from build123d import *

# Parameters (mm, degrees)
PAD_DEPTH       = 70
POCKET_DEPTH    = 22
SKETCH008_W     = 61.659011
SKETCH008_H     = 41.462551
SKETCH008_W_2   = 60.331963
SKETCH008_H_2   = 13.684097
POCKET001_DEPTH = 76
SKETCH003_R     = 1.9
POCKET002_DEPTH = 12
POCKET003_DEPTH = 4
POCKET004_DEPTH = 6
SKETCH009_R     = 1.35
POCKET005_DEPTH = 10
SKETCH030_W     = 28.769002
SKETCH030_H     = 32
POCKET006_DEPTH = 48.001
SKETCH031_W     = 46.619307
SKETCH031_H     = 35.048725
POCKET007_DEPTH = 36
SKETCH032_R     = 1.9
POCKET008_DEPTH = 10
SKETCH013_R     = 1.9
POCKET009_DEPTH = 16
SKETCH010_R     = 1.6
POCKET010_DEPTH = 7
POCKET011_DEPTH = 60.501
POCKET012_DEPTH = 12.001
FILLET_R        = 3
CHAMFER_SIZE    = 3
FILLET001_R     = 5
FILLET002_R     = 9
FILLET003_R     = 0.7
FILLET004_R     = 1
FILLET005_R     = 1
FILLET006_R     = 3
FILLET007_R     = 1
FILLET008_R     = 1
CHAMFER001_SIZE = 13
FILLET009_R     = 1
FILLET010_R     = 16


with BuildPart() as part:
    # Sketch → Pad (new body)
    with BuildSketch(Plane.XY):
        Polygon((0, 0), (44, 0), (44, -60.5), (-14, -60.5), (-14, 0), align=None)
    extrude(amount=PAD_DEPTH)

    # Sketch002 (on Face7 of Pad) → Pocket (cut)
    with BuildSketch(Plane.XY.offset(70)):
        Polygon((32, -6), (32, -65.096024), (-40.783405, -65.096024), (-40.783405, 12.994774), (20, 12.994774), (20, -6), align=None)
    extrude(amount=-POCKET_DEPTH, mode=Mode.SUBTRACT)

    # Sketch008 (on Face3 of Pocket) → Pocket001 (cut)
    with BuildSketch(Plane.YZ.offset(44)):
        with Locations((-36.829505, -1.731275)):
            Rectangle(SKETCH008_W, SKETCH008_H)
        with Locations((-36.165982, 66.842049)):
            Rectangle(SKETCH008_W_2, SKETCH008_H_2)
    extrude(amount=-POCKET001_DEPTH, mode=Mode.SUBTRACT)

    # Sketch003 (on Face6 of Pocket001) → Pocket002 (cut)
    with BuildSketch(Plane.XY.offset(48)):
        with Locations((0, -13)):
            Circle(SKETCH003_R)
        with Locations((0, -57)):
            Circle(SKETCH003_R)
    extrude(amount=-POCKET002_DEPTH, mode=Mode.SUBTRACT)

    # Sketch004 (on Face6 of Pocket002) → Pocket003 (cut)
    with BuildSketch(Plane.XY.offset(48)):
        with BuildLine():
            ThreePointArc((0, -43.125), (8.125, -35), (0, -26.875))
            Line((-25, -26.875), (0, -26.875))
            Line((-25, -43.125), (-25, -26.875))
            Line((0, -43.125), (-25, -43.125))
        make_face()
    extrude(amount=-POCKET003_DEPTH, mode=Mode.SUBTRACT)

    # Sketch018 (on Face22 of Pocket003) → Pocket004 (cut)
    with BuildSketch(Plane.XY.offset(44)):
        with BuildLine():
            ThreePointArc((0, -41.1), (6.1, -35), (0, -28.9))
            Line((0, -28.9), (-50, -28.9))
            Line((-50, -41.1), (-50, -28.9))
            Line((0, -41.1), (-50, -41.1))
        make_face()
    extrude(amount=-POCKET004_DEPTH, mode=Mode.SUBTRACT)

    # Sketch009 (on Face3 of Pocket004) → Pocket005 (cut)
    with BuildSketch(Plane.YZ.offset(44)):
        with Locations((-44, 55)):
            Circle(SKETCH009_R)
        with Locations((-13, 24)):
            Circle(SKETCH009_R)
        with Locations((-13, 55)):
            Circle(SKETCH009_R)
        with Locations((-44, 24)):
            Circle(SKETCH009_R)
    extrude(amount=-POCKET005_DEPTH, mode=Mode.SUBTRACT)

    # Sketch030 (on Face6 of Pocket005) → Pocket006 (cut, through all)
    with BuildSketch(Plane.XY.offset(48)):
        with Locations((-14.384501, -35)):
            Rectangle(SKETCH030_W, SKETCH030_H)
    extrude(amount=-POCKET006_DEPTH, mode=Mode.SUBTRACT)

    # Sketch031 (on Face8 of Pocket006) → Pocket007 (cut)
    with BuildSketch(Plane(origin=(-14, 0, 0), x_dir=(0, -1, 0), z_dir=(-1, 0, 0))):
        with Locations((29.409654, 20.475638)):
            Rectangle(SKETCH031_W, SKETCH031_H)
    extrude(amount=-POCKET007_DEPTH, mode=Mode.SUBTRACT)

    # Sketch032 (on Face8 of Pocket007) → Pocket008 (cut)
    with BuildSketch(Plane(origin=(-14, 0, 0), x_dir=(0, -1, 0), z_dir=(-1, 0, 0))):
        with Locations((12, 44)):
            Circle(SKETCH032_R)
        with Locations((55, 44)):
            Circle(SKETCH032_R)
    extrude(amount=-POCKET008_DEPTH, mode=Mode.SUBTRACT)

    # Sketch013 (on Face21 of Pocket008) → Pocket009 (cut)
    with BuildSketch(Plane(origin=(0, 0, 0), x_dir=(0, -1, 0), z_dir=(-1, 0, 0))):
        with Locations((24, 42)):
            Circle(SKETCH013_R)
        with Locations((46, 42)):
            Circle(SKETCH013_R)
    extrude(amount=-POCKET009_DEPTH, mode=Mode.SUBTRACT)

    # Sketch010 (on Face1 of Pocket009) → Pocket010 (cut)
    with BuildSketch(Plane(origin=(0, 0, 0), x_dir=(-1, 0, 0), z_dir=(0, 1, 0))):
        with Locations((-32, 5)):
            Circle(SKETCH010_R)
        with Locations((-39, 65)):
            Circle(SKETCH010_R)
        with Locations((-25, 65)):
            Circle(SKETCH010_R)
    extrude(amount=-POCKET010_DEPTH, mode=Mode.SUBTRACT)

    # Sketch033 (on Face1 of Pocket010) → Pocket011 (cut, through all)
    with BuildSketch(Plane(origin=(0, 0, 0), x_dir=(-1, 0, 0), z_dir=(0, 1, 0))):
        Polygon((21.995766, 41.653675), (-34.908054, -9.830728), (21.995766, -12.411399), align=None)
    extrude(amount=-POCKET011_DEPTH, mode=Mode.SUBTRACT)

    # Sketch034 (on Face30 of Pocket011) → Pocket012 (cut, through all)
    with BuildSketch(Plane(origin=(32, 0, 0), x_dir=(0, -1, 0), z_dir=(-1, 0, 0))):
        with BuildLine():
            ThreePointArc((15.5, 67.5), (21.211418, 53.711418), (35, 48))
            Line((35, 48), (74.47, 48))
            Line((74.47, 67.5), (74.47, 48))
            Line((15.5, 67.5), (74.47, 67.5))
        make_face()
    extrude(amount=-POCKET012_DEPTH, mode=Mode.SUBTRACT)

    # Fillet
    fillet_edges = [part.edges().sort_by_distance(p)[0] for p in [
        (38, -17, 60),
    ]]
    fillet(fillet_edges, radius=FILLET_R)

    # Chamfer
    chamfer_edges = [part.edges().sort_by_distance(p)[0] for p in [
        (44, -3, 70),
        (20, -3, 70),
    ]]
    chamfer(chamfer_edges, length=CHAMFER_SIZE)

    # Fillet001
    fillet001_edges = [part.edges().sort_by_distance(p)[0] for p in [
        (41, -3, 70),
        (23, -3, 70),
        (20, -3, 67),
    ]]
    fillet(fillet001_edges, radius=FILLET001_R)

    # Fillet002
    fillet002_edges = [part.edges().sort_by_distance(p)[0] for p in [
        (24.042511, -3, 0),
        (3.042509, -56.609654, 19),
    ]]
    fillet(fillet002_edges, radius=FILLET002_R)

    # Fillet003
    fillet003_edges = [part.edges().sort_by_distance(p)[0] for p in [
        (4, -6.1, 38),
        (4, -52.719307, 38),
    ]]
    fillet(fillet003_edges, radius=FILLET003_R)

    # Fillet004
    fillet004_edges = [part.edges().sort_by_distance(p)[0] for p in [
        (-7, -19, 38),
        (-7, -51, 38),
    ]]
    fillet(fillet004_edges, radius=FILLET004_R)

    # Fillet005
    fillet005_edges = [part.edges().sort_by_distance(p)[0] for p in [
        (-7, -51, 48),
        (-7, -19, 48),
    ]]
    fillet(fillet005_edges, radius=FILLET005_R)

    # Fillet006
    fillet006_edges = [part.edges().sort_by_distance(p)[0] for p in [
        (-14, -56.609654, 34.419411),
        (-14, -3.05, 34.419411),
    ]]
    fillet(fillet006_edges, radius=FILLET006_R)

    # Fillet007
    fillet007_edges = [part.edges().sort_by_distance(p)[0] for p in [
        (35.754846, 0, 0),
    ]]
    fillet(fillet007_edges, radius=FILLET007_R)

    # Fillet008
    fillet008_edges = [part.edges().sort_by_distance(p)[0] for p in [
        (25.254845, -60.5, 19),
    ]]
    fillet(fillet008_edges, radius=FILLET008_R)

    # Chamfer001
    chamfer001_edges = [part.edges().sort_by_distance(p)[0] for p in [
        (22, -29.409654, 19),
    ]]
    chamfer(chamfer001_edges, length=CHAMFER001_SIZE)

    # Fillet009
    fillet009_edges = [part.edges().sort_by_distance(p)[0] for p in [
        (35.754846, -6, 0),
    ]]
    fillet(fillet009_edges, radius=FILLET009_R)

    # Fillet010
    fillet010_edges = [part.edges().sort_by_distance(p)[0] for p in [
        (20, -3, 48),
    ]]
    fillet(fillet010_edges, radius=FILLET010_R)


solid = part.part
CAD build for the part. Positions are in the model's coordinates, mm. A direction names the side the tool comes from. Round coordinates to 2 decimals unless told otherwise and drop trailing zeros. Write each loop counter-clockwise with the first axis right and the second up, starting at its lowest first coordinate (ties: lowest second). Pieces come first, ordered by that corner, then holes. Notation, with made-up numbers: M 57.25,49 L 90.25,49 A12 ccw 90.25,54 Z; hole C 47,41.5 d3. An arc over 180 degrees is marked long. Put each result on its own line as item: value. Start each with the question number.
1) Saw through at B-B, the plane y = -31.5. Write the cut outline in (x, z).
2) Pull direction Y, two halves, no side cores. Call faces 5 (the cylindrical face through (12.588, -5.715, 10.769)), 6 (the flat face through (32, -14, 53)), 7 (the cylindrical face through (8.123, -35.179, 46.028)): pulls with the +Y half, pulls with the -Y half, needs draft (parallel to the pull), parting line crosses it, or undercut.
3) Pin check, flat tips, straight feed: pin 1 Ø8 at (y, z) = (-46, 44) entering from -X; pin 2 Ø2 at (y, z) = (-13, 24) entering from -X; pin 3 Ø1 at (x, y) = (38, -30.5) entering from -Z; pin 4 Ø3 at (x, z) = (39, 65) entering from -Y. Stop position of each tip, or through.
4) Drill centre lines: probe 1 along Z at (x, y) = (38.25, -13); probe 2 along Z at (x, y) = (39, -4.25); probe 3 along Z at (x, y) = (-11, -12). Where is each one in solid material? Low to high. Write a range as [from, to].
5) Saw through at A-A, the plane z = 55. Write the cut outline in (x, y), and give its area (3 significant figures).
6) 3-axis set-ups, long thin cutter, end or side, ignore diameter. For faces 1 (the flat face through (36, -38, 19)), 2 (the cylindrical face through (39.07, -13.29, 53.68)), 3 (the flat face through (10, -6.1, 28)), 4 (the flat face through (24, -6, 57)): which of +Z, -Z, +X, -X, +Y, -Y reach the whole face in a straight line?
7) Saw through at D-D, the plane y = -24. Write the cut outline in (x, z).
8) Saw through at C-C, the plane x = 12. Count the separate pieces of the cut face and the enclosed holes in it, and give its area (3 significant figures).
Resolved:
1. outline: M 5,38 L 22,38 L 22,32 L 35,19 L 44,19 L 44,48.32 L 32,48.32 L 32,48 L 7.33,48 L 7.33,44 L 5,44 Z
2. face 5: pulls with the -Y half
2. face 6: needs draft
2. face 7: undercut
3. pin 1: x = 0
3. pin 2: x = 29
3. pin 3: z = 19
3. pin 4: through
4. probe 1: [19, 22.65], [25.35, 53.65], [56.35, 60]
4. probe 2: [0, 63.4], [66.6, 70]
4. probe 3: [38, 42.1], [45.9, 48]
5. outline: M 17.23,-6 L 32,-6 L 32,-20.03 L 44,-20.03 L 44,-14.35 L 34,-14.35 L 34,-11.65 L 44,-11.65 L 44,0 L 17.23,0 Z
5. area: 302 mm²
6. face 1: -Z, +X, -X, -Y
6. face 2: +X
6. face 3: -Z, -X
6. face 4: +Z, -X, -Y
7. outline: M 0,38 L 22,38 L 22,32 L 35,19 L 44,19 L 44,51.4 L 32,51.4 L 32,48 L 0,48 L 0,43.9 L 16,43.9 L 16,40.1 L 0,40.1 Z
8. separate pieces: 1
8. enclosed holes: 2
8. area: 907 mm²
